Build history of the part. All positions in model axes, mm. A direction names the side the tool comes from. Round coordinates to 2 decimals unless told otherwise and drop trailing zeros. Loops run counter-clockwise (first coordinate to the right, second up) from the corner with the lowest first, then second, coordinate; pieces in that order, holes last. Notation, with made-up numbers: (49.5, 43) - (97.5, 43) arc R20 cw to (97.5, 66) - close; hole circle Ø1 at (32, -25.5). An arc over 180 degrees is marked (long way). Put each result on its own line as item: value. Start each with the question number.
Autodesk Inventor part; units mm, degrees
ref_plane "YZ Plane" through (0, 0, 0) normal (1, 0, 0) x (0, 1, 0)
ref_plane "XZ Plane" through (0, 0, 0) normal (0, 1, 0) x (-1, 0, 0)
ref_plane "XY Plane" through (0, 0, 0) normal (0, 0, 1) x (1, 0, 0)
sketch "スケッチ1" plane through (0, 0, 0) normal (0, 0, 1) x (1, 0, 0)
  line L0 (2.75, 1.5877) -> (2.75, -1.5877)
  line L1 (2.75, -1.5877) -> (0, -3.1754)
  line L2 (0, -3.1754) -> (-2.75, -1.5877)
  line L3 (-2.75, -1.5877) -> (-2.75, 1.5877)
  line L4 (-2.75, 1.5877) -> (0, 3.1754)
  line L5 (0, 3.1754) -> (2.75, 1.5877)
  point P0 (0, 0)
  point P1 (0, 0)
  dimension "d0" = 5.5
extrude "押し出し1" add sketch "スケッチ1" along normal blind 25
sketch "スケッチ2" plane through (0, 0, 25) normal (0, 0, 1) x (1, 0, 0)
  point P0 (0, 0)
  point P1 (0, 0)
hole "穴1" at (0, 0, 25) direction (0, 0, -1) diameter 2.459 depth 6
mirror "ミラー1" about plane through (0, 0, 0) normal (0, 0, -1) of "押し出し1", "穴1"
properties part number "ASU-340" material "ステンレス鋼 AISI 304"
Item 1: Slice it at C-C (y = 2.25). Give the cut face in (x, z).
Item 2: Slice it at A-A (y = 0). Give the cut face in (x, z), plus the area to 3 significant figures.
Item 3: Drill centre lines: probe 1 along X at (y, z) = (0, 20.3); probe 2 along Y at (x, z) = (0, 22.55); probe 3 along Y at (x, z) = (-0.1, -20.5). Where is each one in solid material? Low to high. Write a range as [from, to].
Item 4: Drop flat-ended pins along their axis: pin 1 Ø1.2 at (x, y) = (0, 0) entering from -Z; pin 2 Ø1.5 at (x, z) = (2, 13.5) entering from -Y. Give the stop position or say it passes through.
Item 5: Two-plate mould, pull along Y, no slides. Class faces 4 (the cylindrical face through (-0.748, 0.976, -21.958)), 5 (the flat face through (0, -1.4, 25)), 6 (the flat face through (1.36, -2.39, 0.35)): pulls with the +Y half, pulls with the -Y half, needs draft (parallel to the pull), parting line crosses it, or undercut.
Item 6: Slice it at B-B (z = 15). Give the cut face in (x, y).
Item 7: Which spindle directions (+Z, -Z, +X, -X, +Y, -Y) get a long thin tool onto all of the face, cutting with end or side? Do faces 1 (the cylindrical face through (0.748, 0.976, 21.958)), 2 (the flat face through (-2.75, 0, 0)), 3 (the flat face through (0, 0, -19)). Say none if no direction does.
Computed values:
1. outline: (-1.6, -25) - (1.6, -25) - (1.6, 25) - (-1.6, 25) - close
2. outline: (-2.75, -25) - (-1.23, -25) - (-1.23, -19) - (1.23, -19) - (1.23, -25) - (2.75, -25) - (2.75, 25) - (1.23, 25) - (1.23, 19) - (-1.23, 19) - (-1.23, 25) - (-2.75, 25) - close
2. area: 245 mm^2
3. probe 1: x = [-2.75, -1.23], [1.23, 2.75]
3. probe 2: y = [-3.18, -1.23], [1.23, 3.18]
3. probe 3: y = [-3.12, -1.23], [1.23, 3.12]
4. pin 1: stops at z = -19
4. pin 2: stops at y = -2.45
5. face 4: undercut
5. face 5: needs draft
5. face 6: pulls with the -Y half
6. outline: (-2.75, -1.59) - (0, -3.18) - (2.75, -1.59) - (2.75, 1.59) - (0, 3.18) - (-2.75, 1.59) - close
7. face 1: +Z
7. face 2: +Z, -Z, -X, +Y, -Y
7. face 3: -Z
